Autodesk Inventor part; units mm, degrees
ref_plane "YZ Plane" through (0, 0, 0) normal (1, 0, 0) x (0, 1, 0)
ref_plane "XZ Plane" through (0, 0, 0) normal (0, 1, 0) x (-1, 0, 0)
ref_plane "XY Plane" through (0, 0, 0) normal (0, 0, 1) x (1, 0, 0)
sketch "Sketch1" plane through (0, 0, 0) normal (0, 1, 0) x (-1, 0, 0)
  line L0 (0, 0) -> (25.4, 0)
  line L1 (25.4, 0) -> (25.4, -25.4)
  line L2 (25.4, -25.4) -> (0, -25.4)
  line L3 (0, -25.4) -> (0, 0)
  line L4 (1.5875, -23.8125) -> (23.8125, -23.8125)
  line L5 (23.8125, -23.8125) -> (23.8125, -1.5875)
  line L6 (23.8125, -1.5875) -> (1.5875, -1.5875)
  line L7 (1.5875, -1.5875) -> (1.5875, -23.8125)
  dimension "d0" = 25.4
  dimension "d1" = 25.4
  dimension "d2" = 1.5875
extrude "Extrusion1" add sketch "Sketch1" along normal blind 406.4
sketch "Sketch2" plane through (0, 0, 0) normal (1, 0, 0) x (0, 0, -1)
  line L0 (25.4, 0) -> (25.4, 406.4)
  line L1 (25.4, 0) -> (0, 54.4705)
  line L2 (0, 0) -> (0, 406.4)
  line L3 (0, 54.4705) -> (0, 0)
  line L4 (0, 0) -> (25.4, 0)
  dimension "d5" = 25
extrude "Extrusion2" cut sketch "Sketch2" against normal blind 25.4
sketch "Sketch3" plane through (0, 406.4, 0) normal (1, 0, 0) x (0, 0, -1)
  circle A0 centre (12.7, -12.7) radius 3.3734
  line L0 (0, 0) -> (25.4, 0)
  line L1 (0, -351.9295) -> (0, 0)
  circle A1 centre (12.7, -38.1) radius 3.3734
  point P0 (0, -406.4)
  dimension "d8" = 6.7469
  dimension "d9" = 12.7
  dimension "d10" = 12.7
  dimension "d11" = 6.7469
  dimension "d12" = 12.7
  dimension "d13" = 38.1
extrude "Extrusion3" cut sketch "Sketch3" against normal blind 25.4
sketch "Sketch4" plane through (0, 406.4, 0) normal (1, 0, 0) x (0, 0, -1)
  circle A0 centre (12.7, -152.4) radius 3.3734
  line L0 (0, 0) -> (25.4, 0)
  circle A1 centre (12.7, -127) radius 3.3734
  circle A2 centre (12.7, -101.6) radius 3.3734
  line L1 (0, -351.9295) -> (0, 0)
  circle A3 centre (12.7, -247.65) radius 3.3734
  circle A4 centre (12.7, -222.25) radius 3.3734
  circle A5 centre (12.7, -273.05) radius 3.3734
  line L2 (12.7, -273.05) -> (12.7, -222.25) construction
  line L3 (25.4, -406.4) -> (25.4, 0) construction
  point P0 (0, -406.4)
  dimension "d16" = 6.7469
  dimension "d17" = 152.4
  dimension "d18" = 6.7469
  dimension "d19" = 25.4
  dimension "d20" = 6.7469
  dimension "d21" = 12.7
  dimension "d22" = 12.7
  dimension "d23" = 12.7
  dimension "d24" = 25.4
  dimension "d25" = 6.7469
  dimension "d26" = 25.4
  dimension "d27" = 25.4
  dimension "d28" = 12.7
  dimension "d30" = 273.05
extrude "Extrusion4" cut sketch "Sketch4" against normal blind 25.4
sketch "Sketch5" plane through (-25.4, 406.4, -25.4) normal (-1, 0, 0) x (0, 0, 1)
  line L0 (25.4, -351.9295) -> (25.4, 0)
  line L1 (0, -406.4) -> (0, 0)
  point P0 (25.4, -406.4)
  point P1 (0, -351.9295)
properties part number "top" material "Aluminum 6061"
Check sheet for the modelled part. Datum: model origin and axes. Units: mm. A direction names the side the tool comes from. Give positions to 0.01 mm unless a question says otherwise; leave off trailing zeros. Loops run counter-clockwise (first coordinate to the right, second up) from the corner with the lowest first, then second, coordinate; pieces in that order, holes last. Notation, with made-up numbers: M 79.5,33 L 109.5,33 A19 cw 109.5,65 Z; hole C 69,45 d8. An arc over 180 degrees is marked long. Answer as CSV lines item,"result".
Item 1: Sectioned sample at D-D, the plane y = 39. Enter the section's corners in (x, z), then the cut area to 3 significant figures.
Reply:
outline,"M -25.4,-25.4 L 0,-25.4 L 0,-7.21 L -1.59,-7.21 L -1.59,-23.81 L -23.81,-23.81 L -23.81,-7.21 L -25.4,-7.21 Z"
area,"93.0 mm^2"
Item 2: Sectioned sample at A-A, the plane x = -17.25. Enter the section's corners in (y, z).
Reply:
outline,"M 0,-25.4 L 406.4,-25.4 L 406.4,-23.81 L 3.4,-23.81 Z; M 51.07,-1.59 L 406.4,-1.59 L 406.4,0 L 54.47,0 Z"
Item 3: Set-up check for faces 1 (the face through (-23.812, 202, -13)), 2 (the face through (-0.783, 180.857, -11.969)): record each of +Z, -Z, +X, -X, +Y, -Y from which the full face is reachable in a straight line by a thin tool's end or side.
Reply:
face 1,"+Y, -Y"
face 2,"+X, -X"
Item 4: Draft check along Z on faces 3 (the face through (-13, 228, 0)), 4 (the face through (-1, 406.4, -13)), 5 (the face through (-0.783, 130.057, -11.969)). Enter one of: pulls with the +Z half, pulls with the -Z half, needs draft (parallel to the pull), parting line crosses it, or undercut.
Reply:
face 3,"pulls with the +Z half"
face 4,"needs draft"
face 5,"undercut"
Item 5: Sectioned sample at C-C, the plane y = 148.5. Enter the section's corners in (x, z).
Reply:
outline,"M -25.4,-25.4 L 0,-25.4 L 0,0 L -25.4,0 Z; hole M -23.81,-23.81 L -1.59,-23.81 L -1.59,-1.59 L -23.81,-1.59 Z"
Item 6: Sectioned sample at B-B, the plane y = 279.4. Enter the section's corners in (x, z).
Reply:
outline,"M -25.4,-25.4 L 0,-25.4 L 0,-16.07 L -1.59,-16.07 L -1.59,-23.81 L -23.81,-23.81 L -23.81,-16.07 L -25.4,-16.07 Z; M -25.4,-9.33 L -23.81,-9.33 L -23.81,-1.59 L -1.59,-1.59 L -1.59,-9.33 L 0,-9.33 L 0,0 L -25.4,0 Z"
Item 7: Scan lines: L1, parallel to Z at x = -12.5, y = 113.5; L2, parallel to Z at x = -0.8, y = 254. Record each from-to range of solid material in increasing order.
Reply:
L1,"-25.4 to -23.81, -1.59 to 0"
L2,"-25.4 to -16.07, -9.33 to 0"
